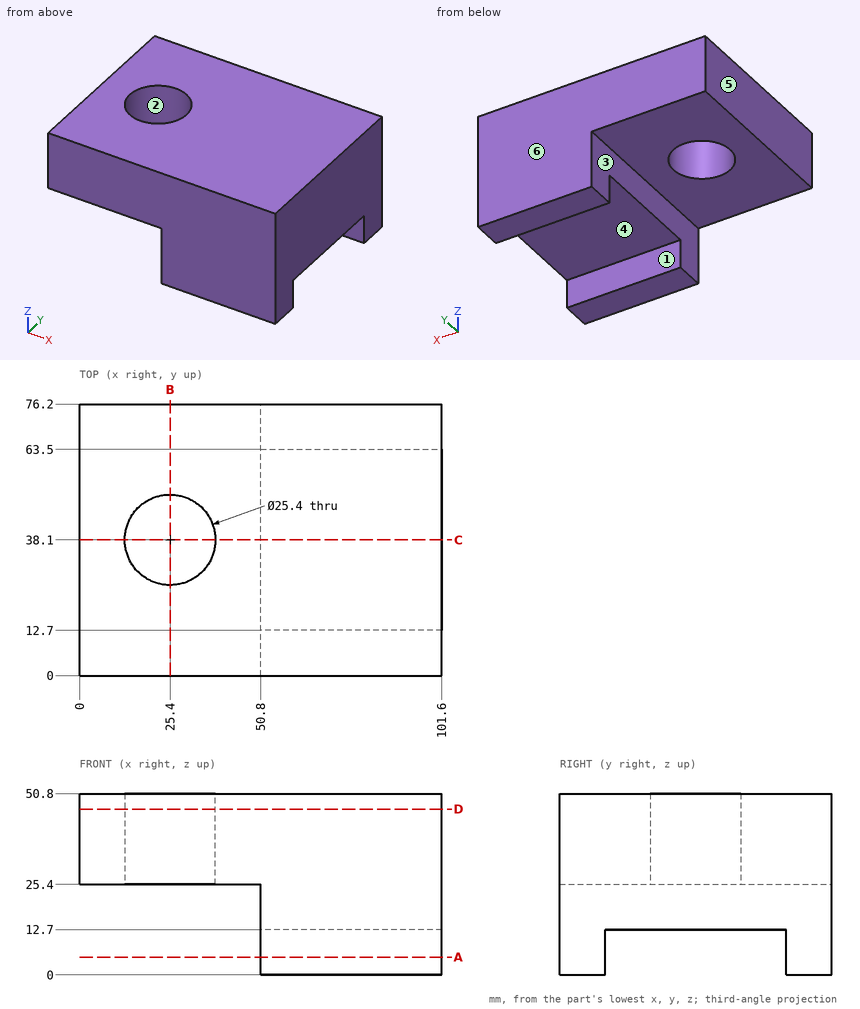
Drawing for the job (mm, zero at the part's lowest x, y, z). A direction names the side the tool comes from. Coordinates: 2 decimals unless noted, no trailing zeros. Order: outer loops, then holes, each group sorted by start corner. A loop starts at its lowest first (then second) coordinate and runs counter-clockwise, first axis right, second up. Notation, with made-up numbers: (18.5, 40) - (29.5, 40) arc R21 ccw to (29.5, 45) - close; hole circle Ø9 at (-38, 21). An arc over 180 degrees is marked (long way). Use a Markdown table: item, result. Add a question column.
(1) Flat gauge pins, fed straight in: pin 1 (3 mm diameter, centred on x = 56.5, y = 25.5, fed in from -Z); pin 2 (20.5 mm diameter, centred on y = 21.5, z = 8, fed in from -X). Where does each tip first touch, or does it go through?
(2) Pull direction Y, two halves, no side cores. Call the marked faces 4, 5 and 6: +Y half, -Y half, draft (parallel to the pull), parting line (faces both ways), or undercut.
(3) Drill centre lines: line 1 along Y through (x, z) = (25.4, 39.5); line 2 along X through (y, z) = (38.1, 39.5); line 3 along Y through (x, z) = (55.5, 6.5). Where is each one in solid material? Low to high. Write a range as [from, to].
(4) Saw through at C-C (y = 38.1). Give the cut face in (x, z).
(5) Saw through at D-D (z = 46.5). Give the cut face in (x, y), then the cut area to 3 significant figures.
(6) Which spindle directions (+Z, -Z, +X, -X, +Y, -Y) get a long thin tool onto all of the face, cutting with end or side? Do the marked faces 1, 2 and 3. Say none if no direction does.
(7) Saw through at A-A (z = 5). Give the cut face in (x, y).
(8) Saw through at B-B (x = 25.4). Give the cut face in (y, z).
Solved:
| question | item | result |
|---|---|---|
| 1 | pin 1 | stops at z = 12.7 |
| 1 | pin 2 | stops at x = 50.8 |
| 2 | face 4 | undercut |
| 2 | face 5 | draft |
| 2 | face 6 | +Y half |
| 3 | line 1 | y = [0, 25.4], [50.8, 76.2] |
| 3 | line 2 | x = [0, 12.7], [38.1, 101.6] |
| 3 | line 3 | y = [0, 12.7], [63.5, 76.2] |
| 4 | outline | (0, 25.4) - (12.7, 25.4) - (12.7, 50.8) - (0, 50.8) - close; (38.1, 25.4) - (50.8, 25.4) - (50.8, 12.7) - (101.6, 12.7) - (101.6, 50.8) - (38.1, 50.8) - close |
| 5 | outline | (0, 0) - (101.6, 0) - (101.6, 76.2) - (0, 76.2) - close; hole circle Ø25.4 at (25.4, 38.1) |
| 5 | area | 7,240 mm² |
| 6 | face 1 | -Z, +X, -X |
| 6 | face 2 | +Z, -Z |
| 6 | face 3 | -Z, -X, +Y, -Y |
| 7 | outline | (50.8, 0) - (101.6, 0) - (101.6, 12.7) - (50.8, 12.7) - close; (50.8, 63.5) - (101.6, 63.5) - (101.6, 76.2) - (50.8, 76.2) - close |
| 8 | outline | (0, 25.4) - (25.4, 25.4) - (25.4, 50.8) - (0, 50.8) - close; (50.8, 25.4) - (76.2, 25.4) - (76.2, 50.8) - (50.8, 50.8) - close |
